from build123d import *

# Parameters (mm, degrees)
SKETCH1_W                 = 12.7
SKETCH1_H                 = 127
BOSS_EXTRUDE1_DEPTH       = 6.35
SKETCH3_W                 = 12.7
SKETCH3_H                 = 12.7
BOSS_EXTRUDE2_DEPTH       = 6.35
SKETCH4_R                 = 3.175
CUT_EXTRUDE1_DEPTH        = 66.068137364
F_4_40_TAPPED_HOLE1_D     = 2.2606
SKETCH6_OUTSIDE_W         = 40.352
SKETCH6_OUTSIDE_H         = 154.652
SKETCH6_OUTSIDE_R         = 330.2
SKETCH6_OUTSIDE_R_2       = 2.5796875
CUT_EXTRUDE3_DEPTH        = 66.068137364
F_6_32_TAPPED_HOLE1_D     = 2.7051
F_6_32_TAPPED_HOLE1_DEPTH = 6.349
F_6_32_TAPPED_HOLE1_TIP   = 0.81269403


with BuildPart() as part:
    # Sketch1 → Boss-Extrude1 (new body)
    with BuildSketch(Plane.XY):
        Rectangle(SKETCH1_W, SKETCH1_H)
    extrude(amount=BOSS_EXTRUDE1_DEPTH)

    # Sketch3 → Boss-Extrude2 (add)
    with BuildSketch(Plane.XY.offset(6.35)):
        with Locations((0, 57.15)):
            Rectangle(SKETCH3_W, SKETCH3_H)
    extrude(amount=BOSS_EXTRUDE2_DEPTH)

    # Sketch4 → Cut-Extrude1 (cut, through all)
    with BuildSketch(Plane(origin=(0, 0, 0), x_dir=(-1, 0, 0), z_dir=(0, 0, -1))):
        with Locations((0, -12.7)):
            Circle(SKETCH4_R)
    extrude(amount=-CUT_EXTRUDE1_DEPTH, mode=Mode.SUBTRACT)

    # #4-40 Tapped Hole1 (through all)
    with Locations(Plane(origin=(0, -57.15, 0), x_dir=(-1, 0, 0), z_dir=(0, 0, -1))):
        with Locations((0, 0)):
            Hole(F_4_40_TAPPED_HOLE1_D / 2)

    # Sketch6 outside → Cut-Extrude3 (cut, through all)
    # profile 1 of 2: a face of its own
    with BuildSketch(Plane.XY.offset(12.7)):
        Rectangle(SKETCH6_OUTSIDE_W, SKETCH6_OUTSIDE_H)
        with Locations((0, 57.15)):
            Circle(SKETCH6_OUTSIDE_R, mode=Mode.SUBTRACT)
    # profile 2 of 2: a face of its own
    with BuildSketch(Plane.XY.offset(12.7)):
        with Locations((0, 57.15)):
            Circle(SKETCH6_OUTSIDE_R_2)
    extrude(amount=-CUT_EXTRUDE3_DEPTH, mode=Mode.SUBTRACT)

    # #6-32 Tapped Hole1
    with Locations(Plane.ZY.offset(6.35)):
        with Locations((3.175, -12.7)):
            Hole(F_6_32_TAPPED_HOLE1_D / 2, depth=F_6_32_TAPPED_HOLE1_DEPTH)
            with Locations((0, 0, -(F_6_32_TAPPED_HOLE1_DEPTH + F_6_32_TAPPED_HOLE1_TIP / 2))):  # 118° drill point
                Cone(0, F_6_32_TAPPED_HOLE1_D / 2, F_6_32_TAPPED_HOLE1_TIP, mode=Mode.SUBTRACT)


solid = part.part
Design review of the part built by this model. Coordinates are the model's own, in mm. A direction names the side the tool comes from. Give positions to 0.01 mm unless a question says otherwise; leave off trailing zeros. Write each loop counter-clockwise with the first axis right and the second up, starting at its lowest first coordinate (ties: lowest second). Pieces come first, ordered by that corner, then holes. Notation, with made-up numbers: M -5.5,21 L 5.5,21 A11 cw 5.5,30 Z; hole C 88.5,82.25 d6. An arc over 180 degrees is marked long. Answer as a JSON object with one key per item and string values. Group by question number.
1) Mouldability with a two-part tool opening along X and no side actions: class faces 1 (the face through (0, 1, 0)), 2 (the face through (3.17, -12.56, 3.13)), 3 (the face through (-6.35, -1, 3)), 4 (the face through (6.35, -1, 3)) as released by +X, released by -X, zero draft, split by the parting line, or undercut.
2) We need section C-C (y = -12.7). Give the boundary of the cut face in (x, z) (3 decimals).
3) Clearance check with flat-ended pins moving along their axes: pin 1 Ø4 at (x, y) = (3, -28.5) entering from +Z; pin 2 Ø3 at (x, z) = (1, 10.5) entering from -Y; pin 3 Ø6 at (x, y) = (0, 57.15) entering from -Z; pin 4 Ø2 at (y, z) = (-12.7, 3.175) entering from -X. State where each tip first meets the part, or that it passes through.
4) We need section A-A (y = 57.15). Give the boundary of the cut face in (x, z), and give its area (3 significant figures).
5) We need section B-B (x = 0). Give the boundary of the cut face in (y, z) (3 decimals).
6) For line 1 along Y through (x, z) = (0, 1.75) (3 decimals); line 2 along Y through (x, z) = (1.25, 4.5); line 3 along Z through (x, y) = (-4.7, -12.7), list the stretches that pass through material, from the lowest coordinate up.
7) Tool access review of faces 5 (the face through (-4.59, -11.36, 3.35)), 6 (the face through (0, 50.8, 9)), 7 (the face through (0, -63.5, 3)): name each direction out of +Z, -Z, +X, -X, +Y, -Y from which nothing blocks a thin tool from reaching the whole face with its end or side.
8) We need section D-D (y = -57.15). Give the boundary of the cut face in (x, z).
Answer key:
{
 "1": {"face 1": "zero draft", "face 2": "undercut", "face 3": "released by -X", "face 4": "released by +X"},
 "2": {"outline": "M -6.35,0 L -3.175,0 L -3.175,1.822 L -6.35,1.822 Z; M -6.35,4.528 L -3.175,4.528 L -3.175,6.35 L -6.35,6.35 Z; M 3.175,0 L 6.35,0 L 6.35,6.35 L 3.175,6.35 Z"},
 "3": {"pin 1": "stops at z = 6.35", "pin 2": "stops at y = 50.8", "pin 3": "stops at z = 0", "pin 4": "stops at x = 3.01"},
 "4": {"outline": "M -6.35,0 L -2.58,0 L -2.58,12.7 L -6.35,12.7 Z; M 2.58,0 L 6.35,0 L 6.35,12.7 L 2.58,12.7 Z", "area": "95.8 mm²"},
 "5": {"outline": "M -63.5,0 L -58.28,0 L -58.28,6.35 L -63.5,6.35 Z; M -56.02,0 L -15.875,0 L -15.875,6.35 L -56.02,6.35 Z; M -9.525,0 L 54.57,0 L 54.57,12.7 L 50.8,12.7 L 50.8,6.35 L -9.525,6.35 Z; M 59.73,0 L 63.5,0 L 63.5,12.7 L 59.73,12.7 Z"},
 "6": {"line 1": "y = -63.5 to -58.28, -56.02 to -15.875, -9.525 to 54.57, 59.73 to 63.5", "line 2": "y = -63.5 to -15.62, -9.78 to 54.89, 59.41 to 63.5", "line 3": "z = 0 to 1.82, 4.53 to 6.35"},
 "7": {"face 5": "-X", "face 6": "+Z, +X, -X, -Y", "face 7": "+Z, -Z, +X, -X, -Y"},
 "8": {"outline": "M -6.35,0 L -1.13,0 L -1.13,6.35 L -6.35,6.35 Z; M 1.13,0 L 6.35,0 L 6.35,6.35 L 1.13,6.35 Z"}
}
